from build123d import *

# Parameters (mm, degrees)
F1_DEPTH     = 40
F2_T1_DEPTH  = 26.5951332913
F2_T6_DEPTH  = 26.5
F2_T11_DEPTH = 26.5


# Not quite as in the source:
# - a fillet or chamfer that OpenCascade refuses, or shapes differently, is made with other operations: its cross-section is extruded or revolved along the edge and cut away or added


with BuildPart() as f1:
    # F0 (on Right) → F1 (new body, symmetric)
    with BuildSketch(Plane.YZ):
        with BuildLine():
            Line((-7.5, 5), (-7.5, 0))
            ThreePointArc((-7.5, 0), (-1.2951320089, -7.3873292251), (7.0527021545, -2.5513510773))
            Line((7.0527021545, -2.5513510773), (44.82801842, 101.87099079))
            ThreePointArc((44.82801842, 101.87099079), (50, 105.5), (55.17198158, 101.87099079))
            Line((55.17198158, 101.87099079), (94.7374969044, -7.5))
            Line((94.7374969044, -7.5), (96.3326301957, -7.5))
            Line((96.3326301957, -7.5), (56.5825220109, 102.3812610054))
            ThreePointArc((56.5825220109, 102.3812610054), (50, 107), (43.4174779891, 102.3812610054))
            Line((43.4174779891, 102.3812610054), (5.6421617236, -2.0410808618))
            ThreePointArc((5.6421617236, -2.0410808618), (-1.0361056071, -5.9098633801), (-6, 0))
            Line((-6, 0), (-6, 5))
            Line((-6, 5), (-7.5, 5))
        make_face()
    extrude(amount=F1_DEPTH, both=True)

    # F2: fillet of radius 5 on 4 edges, made by hand

    # F2_s2 → F2_t1 (cut)
    with BuildSketch(Plane.XZ.offset(-108.8326301957)):
        with BuildLine():
            ThreePointArc((-35, -7.5), (-38.5355339059, -6.0355339059), (-40, -2.5))
            Line((-40, -2.5), (-40, -7.5))
            Line((-40, -7.5), (-35, -7.5))
        make_face()
        with BuildLine():
            ThreePointArc((35, -7.5), (38.5355339059, -6.0355339059), (40, -2.5))
            Line((40, -2.5), (40, -7.5))
            Line((40, -7.5), (35, -7.5))
        make_face()
    extrude(amount=F2_T1_DEPTH, mode=Mode.SUBTRACT)


with BuildPart() as f2_tool4:
    # F2_s5 → F2_t6 (new body)
    with BuildSketch(Plane.XZ.offset(-6.5)):
        with BuildLine():
            ThreePointArc((35, 5), (38.5355339059, 3.5355339059), (40, 0))
            Line((40, 0), (40, 5))
            Line((40, 5), (35, 5))
        make_face()
    extrude(amount=F2_T6_DEPTH)

    split(bisect_by=Plane(origin=(0, 5.6421617236, -2.0410808618), x_dir=(1, 0, 0), z_dir=(0, -0.9403602873, 0.3401801436)), keep=Keep.TOP)


with BuildPart() as f1_1:
    add(f1.part)

    # F2_t3: cut F2_tool4
    add(f2_tool4.part, mode=Mode.SUBTRACT)


with BuildPart() as f2_tool9:
    # F2_s10 → F2_t11 (new body)
    with BuildSketch(Plane.XZ.offset(-6.5)):
        with BuildLine():
            ThreePointArc((-35, 5), (-38.5355339059, 3.5355339059), (-40, 0))
            Line((-40, 0), (-40, 5))
            Line((-40, 5), (-35, 5))
        make_face()
    extrude(amount=F2_T11_DEPTH)

    split(bisect_by=Plane(origin=(0, 5.6421617236, -2.0410808618), x_dir=(1, 0, 0), z_dir=(0, -0.9403602873, 0.3401801436)), keep=Keep.TOP)


with BuildPart() as f1_2:
    add(f1_1.part)

    # F2_t8: cut F2_tool9
    add(f2_tool9.part, mode=Mode.SUBTRACT)


solid = f1_2.part
Input: part model. Units: mm. Frame: model coordinates. A direction names the side the tool comes from. Round coordinates to 2 decimals unless told otherwise and drop trailing zeros. Loops run counter-clockwise (first coordinate to the right, second up) from the corner with the lowest first, then second, coordinate; pieces in that order, holes last. Notation, with made-up numbers: (15, 71.25) -> (49, 71.25) arc R19 ccw to (49, 104.25) -> close; hole circle Ø9 at (-15, 19). An arc over 180 degrees is marked (long way). Answer as a JSON object with one key per item and string values. Group by question number.
1) Section query B-B on z = 98. Output: boundary loops of the cut face in (x, y), plus the area to 3 significant figures.
2) Section query C-C on x = 29.5. Output: boundary loops of the cut face in (y, z), plus the area to 3 significant figures.
3) Reachability of faces 1 (the cylindrical face through (-38.5, 95.03, -6.07)), 2 (the flat face through (0.56, 74.68, 47.95)), 3 (the flat face through (40, 28, 58)), 4 (the cylindrical face through (38.5, 95.03, -6.07)), 5 (the cylindrical face through (38, -7, 4)) from +Z, -Z, +X, -X, +Y, -Y: full face, straight path, thin tool, end or side. Return the list, or none.
4) Draft query along Y for faces 6 (the cylindrical face through (0.6, 49.9, 105.5)), 7 (the cylindrical face through (1, 50, 107)), 8 (the flat face through (1, -6, 2)), 9 (the cylindrical face through (-38, -7, 4)). Return one class per face: +Y half, -Y half, draft (parallel to the pull), parting line (faces both ways), or undercut.
5) Ray query, L1, parallel to Y at x = -31.5, z = 81.5; L2, parallel to Y at x = 21, z = 89; L3, parallel to Z at x = -2, y = 4. Return the intervals inside material, ascending.
6) Section query A-A on z = 3. Output: boundary loops of the cut face in (x, y).
7) Pin query (flat end, axial travel): pin 1 (1.5 mm diameter, centred on x = 12, z = 9.5, fed in from +Y); pin 2 (6 mm diameter, centred on x = 12, z = 10.5, fed in from -Y); pin 3 (8 mm diameter, centred on x = -15, z = 23.5, fed in from -Y). Return the tip coordinate at first contact, or that it passes through.
8) Section query D-D on y = 0. Output: boundary loops of the cut face in (x, z), plus the area to 3 significant figures.
Reply:
{
 "1": {"outline": "(-40, 41.83) -> (40, 41.83) -> (40, 43.43) -> (-40, 43.43) -> close; (-40, 56.57) -> (40, 56.57) -> (40, 58.17) -> (-40, 58.17) -> close", "area": "255 mm2"},
 "2": {"outline": "(-7.5, 0) arc R7.5 ccw to (7.05, -2.55) -> (44.83, 101.87) arc R5.5 cw to (55.17, 101.87) -> (94.74, -7.5) -> (96.33, -7.5) -> (56.58, 102.38) arc R7 ccw to (43.42, 102.38) -> (5.64, -2.04) arc R6 cw to (-6, 0) -> (-6, 5) -> (-7.5, 5) -> close", "area": "400 mm2"},
 "3": {"face 1": "-Z, -X, +Y", "face 2": "-Z, +X, -X", "face 3": "+Z, -Z, +X, +Y, -Y", "face 4": "-Z, +X, +Y", "face 5": "+Z, +X, -Y"},
 "4": {"face 6": "undercut", "face 7": "parting line", "face 8": "undercut", "face 9": "draft"},
 "5": {"L1": "y = 35.86 to 37.46, 62.54 to 64.14", "L2": "y = 38.58 to 40.17, 59.83 to 61.42", "L3": "z = -6.34 to -4.47"},
 "6": {"outline": "(-40, 7.47) -> (40, 7.47) -> (40, 9.06) -> (-40, 9.06) -> close; (-40, 90.94) -> (40, 90.94) -> (40, 92.53) -> (-40, 92.53) -> close; (-39, -7.5) -> (39, -7.5) -> (39, -6) -> (-39, -6) -> close"},
 "7": {"pin 1": "stops at y = 90.45", "pin 2": "stops at y = 9.09", "pin 3": "stops at y = 13.43"},
 "8": {"outline": "(-40, -7.5) -> (40, -7.5) -> (40, -6) -> (-40, -6) -> close", "area": "120 mm2"}
}
